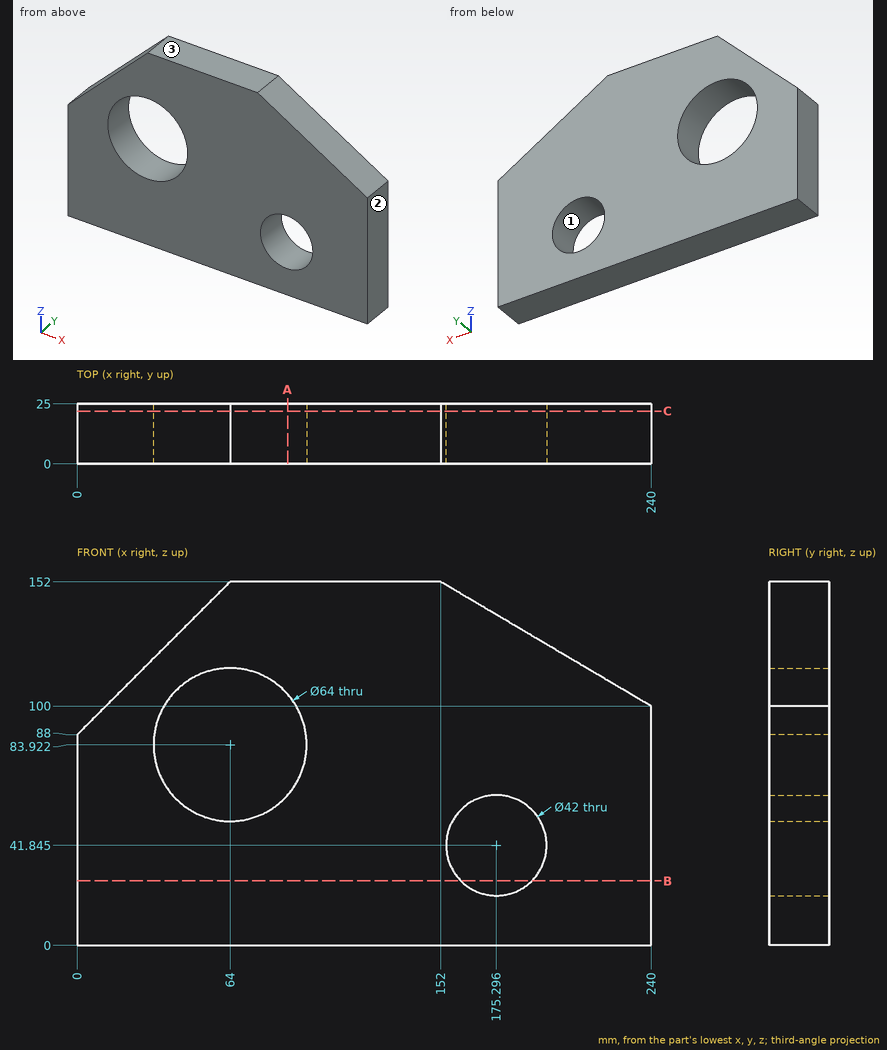
The figure shows three views and two pictorial views of one solid part (mm, origin at its lowest corner). Answer the questions. Give positions to 0.01 mm unless a question says otherwise; leave off trailing zeros. Write each loop counter-clockwise with the first axis right and the second up, starting at its lowest first coordinate (ties: lowest second). Pieces come first, ordered by that corner, then holes. Notation, with made-up numbers: M 13.25,27.5 L 34.25,27.5 A10 cw 34.25,39.5 Z; hole C 26.25,62.25 d10. An arc over 180 degrees is marked long. One line per item, written item: value. Start each with the question number.
(1) Find the intervals of material crossed by line 1 (Z direction, x = 56.5, y = 23.5); line 2 (X direction, y = 16.25, z = 55) (1 decimal); line 3 (X direction, y = 20.5, z = 103) (1 decimal), in increasing order.
(2) Flat-ended cylindrical pins translate along their axes: pin 1 Ø4 at (y, z) = (13.5, 114) entering from +X; pin 2 Ø3 at (y, z) = (22.5, 96.5) entering from -X; pin 3 Ø4 at (y, z) = (18.5, 102.5) entering from +X (1 decimal). Find the tip coordinate at first contact, or state that the pin passes through.
(3) Find section C-C (y = 22). Determine the outline of the cut face in (x, z) (1 decimal).
(4) Find section A-A (x = 88). Determine the outline of the cut face in (y, z) (1 decimal).
(5) Determine the mould class of the marked faces 1, 2 and 3 for opening direction Z: pulls with the +Z half, pulls with the -Z half, needs draft (parallel to the pull), parting line crosses it, or undercut.
(6) Find section B-B (z = 27). Determine the outline of the cut face in (x, y), plus the area to 3 significant figures.
Results below:
1. line 1: z = 0 to 52.81, 115.03 to 144.5
1. line 2: x = 0 to 50.3, 77.7 to 158.9, 191.7 to 240
1. line 3: x = 15 to 38.3, 89.7 to 234.9
2. pin 1: stops at x = 219.69
2. pin 2: stops at x = 7
2. pin 3: stops at x = 239.2
3. outline: M 0,0 L 240,0 L 240,100 L 152,152 L 64,152 L 0,88 Z; hole C 64,83.9 d64; hole C 175.3,41.8 d42
4. outline: M 0,0 L 25,0 L 25,62.8 L 0,62.8 Z; M 0,105.1 L 25,105.1 L 25,152 L 0,152 Z
5. face 1: undercut
5. face 2: needs draft
5. face 3: pulls with the +Z half
6. outline: M 0,0 L 160.44,0 L 160.44,25 L 0,25 Z; M 190.15,0 L 240,0 L 240,25 L 190.15,25 Z
6. area: 5,260 mm^2
